Source: CAD feature listing. Evaluate the final solid. Frame: model axes, mm. A direction names the side the tool comes from. Round coordinates to 2 decimals unless told otherwise and drop trailing zeros. Loops run counter-clockwise (first coordinate to the right, second up) from the corner with the lowest first, then second, coordinate; pieces in that order, holes last.
Item 1: Pull-direction query (X, two-part tool) for faces 4 (the flat face through (0, 1.5, 0)), 5 (the flat face through (27.25, 1, 0)), 6 (the flat face through (-13, 1, 1.25)), 7 (the flat face through (-15.25, 1, -6)); classes: released by +X, released by -X, zero draft, split by the parting line, or undercut.
Item 2: Section query B-B on y = 0.5. Return loops of the section in (x, z), then the cut area to 3 significant figures.
Item 3: Ray query, L1, parallel to X at y = 0.7, z = -2.5; L2, parallel to X at y = 0.8, z = 9.5; L3, parallel to Z at x = -13, y = 0.15. Return the intervals inside material, ascending.
Item 4: Access query for faces 1 (the flat face through (13, 1, -13.25)), 2 (the flat face through (3, 1, 7.25)), 3 (the flat face through (-9, 1, 17.25)). Directions: +Z, -Z, +X, -X, +Y, -Y. A direction counts if a zero-diameter tool reaches every point of the face in a straight line with its end or side. Return the directions, or none.
Item 5: Section query C-C on x = -11. Return loops of the section in (y, z).
Item 6: Section query A-A on z = -1. Return loops of the section in (x, y).
Item 7: Section query D-D on z = 13. Return loops of the section in (x, y), then the cut area to 4 significant figures.
```python
from build123d import *

# Parameters (mm, degrees)
SKETCH1_W           = 54.5
SKETCH1_H           = 34.5
BOSS_EXTRUDE1_DEPTH = 1.5
SKETCH6_W           = 5
SKETCH6_H           = 14.5
CUT_EXTRUDE1_DEPTH  = 2
SKETCH9_W           = 5
SKETCH9_H           = 14.5
CUT_EXTRUDE2_DEPTH  = 2
SKETCH27_W          = 1.5
SKETCH27_H          = 10
CUT_EXTRUDE3_DEPTH  = 2
SKETCH37_W          = 1.5
SKETCH37_H          = 10
CUT_EXTRUDE10_DEPTH = 2


with BuildPart() as part:
    # Sketch1 → Boss-Extrude1 (new body)
    with BuildSketch(Plane(origin=(0, 0, 0), x_dir=(1, 0, 0), z_dir=(0, 1, 0))):
        Rectangle(SKETCH1_W, SKETCH1_H)
    extrude(amount=BOSS_EXTRUDE1_DEPTH)

    # Sketch6 → Cut-Extrude1 (cut)
    with BuildSketch(Plane(origin=(0, 1.5, 0), x_dir=(1, 0, 0), z_dir=(0, 1, 0))):
        with Locations((-12.75, 6)):
            Rectangle(SKETCH6_W, SKETCH6_H)
    extrude(amount=-CUT_EXTRUDE1_DEPTH, mode=Mode.SUBTRACT)

    # Sketch9 → Cut-Extrude2 (cut)
    with BuildSketch(Plane(origin=(0, 1.5, 0), x_dir=(1, 0, 0), z_dir=(0, 1, 0))):
        with Locations((12.75, 6)):
            Rectangle(SKETCH9_W, SKETCH9_H)
    extrude(amount=-CUT_EXTRUDE2_DEPTH, mode=Mode.SUBTRACT)

    # Sketch27 → Cut-Extrude3 (cut)
    with BuildSketch(Plane(origin=(0, 1.5, 0), x_dir=(1, 0, 0), z_dir=(0, 1, 0))):
        with Locations((-21, -12.25)):
            Rectangle(SKETCH27_W, SKETCH27_H)
    extrude(amount=-CUT_EXTRUDE3_DEPTH, mode=Mode.SUBTRACT)

    # Sketch37 → Cut-Extrude10 (cut)
    with BuildSketch(Plane(origin=(0, 1.5, 0), x_dir=(1, 0, 0), z_dir=(0, 1, 0))):
        with Locations((3.5, -12.25)):
            Rectangle(SKETCH37_W, SKETCH37_H)
    extrude(amount=-CUT_EXTRUDE10_DEPTH, mode=Mode.SUBTRACT)


solid = part.part
```
Data:
1. face 4: zero draft
1. face 5: released by +X
1. face 6: undercut
1. face 7: undercut
2. outline: (-27.25, -17.25) - (27.25, -17.25) - (27.25, 17.25) - (4.25, 17.25) - (4.25, 7.25) - (2.75, 7.25) - (2.75, 17.25) - (-20.25, 17.25) - (-20.25, 7.25) - (-21.75, 7.25) - (-21.75, 17.25) - (-27.25, 17.25) - close; hole (-15.25, -13.25) - (-10.25, -13.25) - (-10.25, 1.25) - (-15.25, 1.25) - close; hole (10.25, -13.25) - (15.25, -13.25) - (15.25, 1.25) - (10.25, 1.25) - close
2. area: 1,710 mm2
3. L1: x = -27.25 to -15.25, -10.25 to 10.25, 15.25 to 27.25
3. L2: x = -27.25 to -21.75, -20.25 to 2.75, 4.25 to 27.25
3. L3: z = -17.25 to -13.25, 1.25 to 17.25
4. face 1: +Y, -Y
4. face 2: +Z, +Y, -Y
4. face 3: +Z, +X, -X, +Y, -Y
5. outline: (0, -17.25) - (1.5, -17.25) - (1.5, -13.25) - (0, -13.25) - close; (0, 1.25) - (1.5, 1.25) - (1.5, 17.25) - (0, 17.25) - close
6. outline: (-27.25, 0) - (-15.25, 0) - (-15.25, 1.5) - (-27.25, 1.5) - close; (-10.25, 0) - (10.25, 0) - (10.25, 1.5) - (-10.25, 1.5) - close; (15.25, 0) - (27.25, 0) - (27.25, 1.5) - (15.25, 1.5) - close
7. outline: (-27.25, 0) - (-21.75, 0) - (-21.75, 1.5) - (-27.25, 1.5) - close; (-20.25, 0) - (2.75, 0) - (2.75, 1.5) - (-20.25, 1.5) - close; (4.25, 0) - (27.25, 0) - (27.25, 1.5) - (4.25, 1.5) - close
7. area: 77.25 mm2
